The listing builds one solid part. Answer for the finished solid, in the listing's coordinates (mm). Face numbers are marked on the shaded views. A direction names the side the tool comes from. Give positions to 0.01 mm unless a question says otherwise; leave off trailing zeros. Write each loop counter-clockwise with the first axis right and the second up, starting at its lowest first coordinate (ties: lowest second). Pieces come first, ordered by that corner, then holes. Notation, with made-up numbers: M 43.5,78 L 88.5,78 A10 ccw 88.5,84 Z; hole C 73.5,36.25 d4. An arc over 180 degrees is marked long. Return JSON: item names as keys, results as strings.
from build123d import *

# Parameters (mm, degrees)
SKETCH1_R           = 6.5
BOSS_EXTRUDE1_DEPTH = 6.5
SKETCH2_R           = 1.25
BOSS_EXTRUDE2_DEPTH = 0.5
SKETCH4_R           = 2.5
BOSS_EXTRUDE4_DEPTH = 14
SKETCH5_R           = 0.5
BOSS_EXTRUDE5_DEPTH = 10


with BuildPart() as part:
    # Sketch1 → Boss-Extrude1 (new body)
    with BuildSketch(Plane(origin=(0, 0, 0), x_dir=(1, 0, 0), z_dir=(0, 1, 0))):
        with Locations(Location((0, 0, 0), (0, 0, 90))):
            Circle(SKETCH1_R)
    extrude(amount=BOSS_EXTRUDE1_DEPTH)

    # Sketch2 → Boss-Extrude2 (add)
    with BuildSketch(Plane(origin=(0, 6.5, 0), x_dir=(1, 0, 0), z_dir=(0, 1, 0))):
        with Locations(Location((0, 0, 0), (0, 0, 270))):
            Circle(SKETCH2_R)
    extrude(amount=BOSS_EXTRUDE2_DEPTH)

    # Sketch4 → Boss-Extrude4 (add)
    with BuildSketch(Plane.XY):
        with Locations(Location((0, 3.25, 0), (0, 0, 180))):
            Circle(SKETCH4_R)
    extrude(amount=BOSS_EXTRUDE4_DEPTH)

    # Sketch5 → Boss-Extrude5 (add)
    with BuildSketch(Plane.XY.offset(14)):
        with Locations((0, 3.25)):
            Circle(SKETCH5_R)
    extrude(amount=BOSS_EXTRUDE5_DEPTH)


solid = part.part
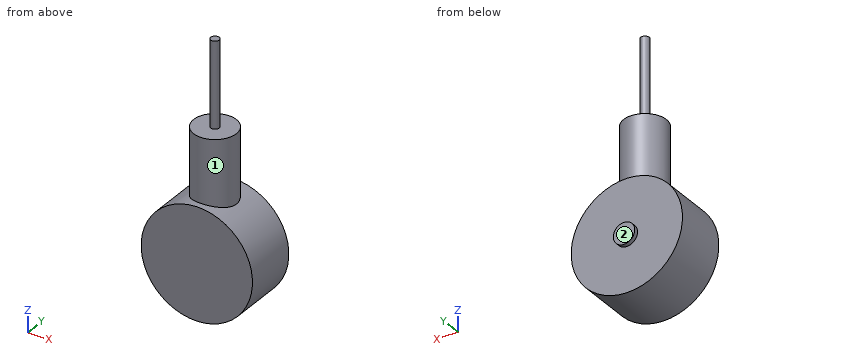
Item 1: A cutting plane is placed at B-B, the plane x = 0. Write down the section's boundary in (y, z), plus the area to 3 significant figures.
Geometry results:
{"outline": "M 0,-6.5 L 6.5,-6.5 L 6.5,-1.25 L 7,-1.25 L 7,1.25 L 6.5,1.25 L 6.5,6.5 L 5.75,6.5 L 5.75,14 L 3.75,14 L 3.75,24 L 2.75,24 L 2.75,14 L 0.75,14 L 0.75,6.5 L 0,6.5 Z", "area": "133 mm2"}
Item 2: Given pin 1 Ø1 at (x, y) = (-5, 1.5) entering from +Z; pin 2 Ø4 at (y, z) = (1, 13) entering from -X; pin 3 Ø3 at (y, z) = (1.5, 4.5) entering from -X, each flat-ended and moving along its own axis, determine where each tip first touches the part or whether it passes through.
Geometry results:
{"pin 1": "stops at z = 4.69", "pin 2": "stops at x = -2.49", "pin 3": "stops at x = -5.77"}
Item 3: A cutting plane is placed at A-A, the plane z = 0. Write down the section's boundary in (x, y), plus the area to 4 significant figures.
Geometry results:
{"outline": "M -6.5,0 L 6.5,0 L 6.5,6.5 L 1.25,6.5 L 1.25,7 L -1.25,7 L -1.25,6.5 L -6.5,6.5 Z", "area": "85.75 mm2"}
Item 4: A cutting plane is placed at D-D, the plane z = 15. Write down the section's boundary in (x, y).
Geometry results:
{"outline": "C 0,3.25 d1"}
Item 5: A cutting plane is placed at C-C, the plane y = 3.25. Write down the section's boundary in (x, z).
Geometry results:
{"outline": "M -2.5,6 A6.5 ccw long 2.5,6 L 2.5,14 L 0.5,14 L 0.5,24 L -0.5,24 L -0.5,14 L -2.5,14 Z"}
Item 6: Find the intervals of material crossed by line 1 (Y direction, x = 2.5, z = -0.5); line 2 (Y direction, x = 0, z = 12); line 3 (X direction, y = 1.75, z = -2), in increasing order.
Geometry results:
{"line 1": "y = 0 to 6.5", "line 2": "y = 0.75 to 5.75", "line 3": "x = -6.18 to 6.18"}
Item 7: Which of the six approach directions +Z, -Z, +X, -X, +Y, -Y give full straight-line access (tool end or side, diameter ignored) to the marked faces 1 and 2?
Geometry results:
{"face 1": "+Z", "face 2": "+Z, -Z, +X, -X, +Y"}
